Design review of the part shown in the three views and the two pictorial views. Dimensions are in mm from the part's minimum x, y and z. A direction names the side the tool comes from. Round coordinates to 2 decimals unless told otherwise and drop trailing zeros. Loops run counter-clockwise (first coordinate to the right, second up) from the corner with the lowest first, then second, coordinate; pieces in that order, holes last. Notation, with made-up numbers: (65.5, 75.5) -> (94.5, 75.5) arc R7 cw to (94.5, 79.5) -> close; hole circle Ø3 at (60.25, 47.25). An arc over 180 degrees is marked (long way). Use a Markdown table: item, result. Add a question column.
1) Mouldability with a two-part tool opening along X and no side actions: class the marked faces 6, 7 and 8 as released by +X, released by -X, zero draft, split by the parting line, or undercut.
2) Insertion check: pin 1 (5 mm diameter, centred on x = 10, z = 7.5, fed in from +Y); pin 2 (4 mm diameter, centred on x = 20.5, y = 6, fed in from -Z); pin 3 (2 mm diameter, centred on y = 14, z = 6.5, fed in from -X); pin 4 (3 mm diameter, centred on x = 20.5, y = 16, fed in from -Z). Each pin has a flat end and moves straight along its axis. Give the tip position at first contact, or say it passes through.
3) Wall thickness on probe 1 along Y at (x, z) = (20.5, 5.5); probe 2 along Z at (x, y) = (5, 6); probe 3 along Y at (x, z) = (18.25, 4.5): over which ranges is each line inside the solid? List them lowest first.
4) Consider section A-A on y = 6. Give the boundary of the cut face in (x, z), plus the area to 3 significant figures.
5) Consider section C-C on x = 5. Give the boundary of the cut face in (y, z).
6) Consider section D-D on x = 20.5. Give the boundary of the cut face in (y, z), plus the area to 3 significant figures.
7) For the marked faces 1, 2, 3, 4 and 5, list the 3-axis set-ups (+Z, -Z, +X, -X, +Y, -Y) from which the entire face can be reached by the end or side of a thin tool; tool diameter is ignored.
8) Consider section B-B on z = 7. State how many separate pieces and enclosed holes the cut face has.
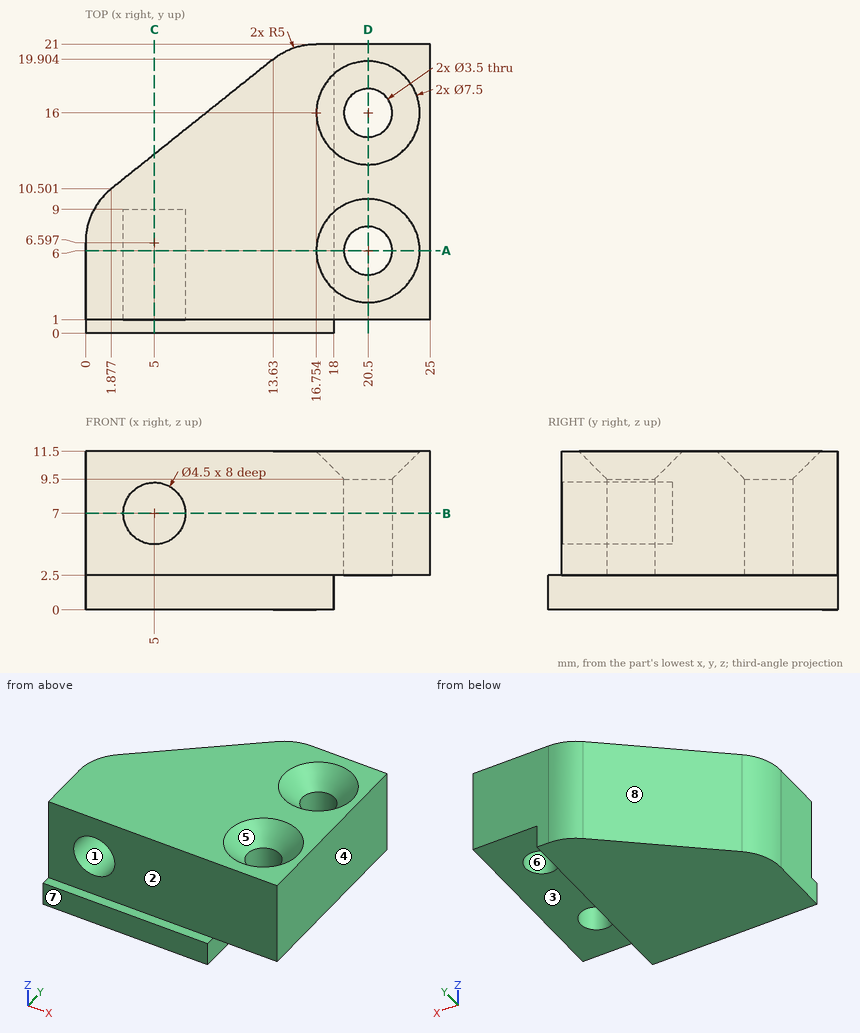
Result set:
| question | item | result |
|---|---|---|
| 1 | face 6 | undercut |
| 1 | face 7 | zero draft |
| 1 | face 8 | released by -X |
| 2 | pin 1 | y = 19 |
| 2 | pin 2 | z = 2.5 |
| 2 | pin 3 | x = 5 |
| 2 | pin 4 | through |
| 3 | probe 1 | 1 to 4.25, 7.75 to 14.25, 17.75 to 21 |
| 3 | probe 2 | 0 to 4.75, 9.25 to 11.5 |
| 3 | probe 3 | 1 to 21 |
| 4 | outline | (0, 0) -> (18, 0) -> (18, 2.5) -> (18.75, 2.5) -> (18.75, 9.5) -> (16.75, 11.5) -> (0, 11.5) -> close; (22.25, 2.5) -> (25, 2.5) -> (25, 11.5) -> (24.25, 11.5) -> (22.25, 9.5) -> close; hole circle Ø4.5 at (5, 7) |
| 4 | area | 219 mm2 |
| 5 | outline | (0, 0) -> (13, 0) -> (13, 11.5) -> (1, 11.5) -> (1, 9.25) -> (9, 9.25) -> (9, 4.75) -> (1, 4.75) -> (1, 2.5) -> (0, 2.5) -> close |
| 6 | outline | (1, 2.5) -> (4.25, 2.5) -> (4.25, 9.5) -> (2.25, 11.5) -> (1, 11.5) -> close; (7.75, 2.5) -> (14.25, 2.5) -> (14.25, 9.5) -> (12.25, 11.5) -> (9.75, 11.5) -> (7.75, 9.5) -> close; (17.75, 2.5) -> (21, 2.5) -> (21, 11.5) -> (19.75, 11.5) -> (17.75, 9.5) -> close |
| 6 | area | 109 mm2 |
| 7 | face 1 | -Y |
| 7 | face 2 | +Z, +X, -X, -Y |
| 7 | face 3 | -Z, +X, +Y, -Y |
| 7 | face 4 | +Z, -Z, +X, +Y, -Y |
| 7 | face 5 | +Z |
| 8 | separate pieces | 1 |
| 8 | enclosed holes | 2 |
